The listing builds one solid part. Answer for the finished solid, in the listing's coordinates (mm). Coordinates: 2 decimals unless noted, no trailing zeros. Order: outer loops, then holes, each group sorted by start corner. A loop starts at its lowest first (then second) coordinate and runs counter-clockwise, first axis right, second up. Notation, with made-up numbers: (9.25, -30) -> (51.25, -30) arc R12 ccw to (51.25, -16) -> close; hole circle Ø8 at (27.5, 55.25). An arc over 180 degrees is marked (long way). Write each question's results on one line, items separated by ' | '. Start each with the question number.
(1) The part is cut by section C-C, the plane x = -32. Give the vertices of the cut face in (y, z).
(2) The part is cut by section A-A, the plane z = 57. Give the vertices of the cut face in (x, y).
(3) Given pin 1 (1.5 mm diameter, centred on x = 1.5, y = -4.5, fed in from -Z); pin 2 (1.5 mm diameter, centred on x = -1.5, y = -4, fed in from +Z); pin 3 (2 mm diameter, centred on x = -16.5, z = 46.5, fed in from -Y); pin 4 (4 mm diameter, centred on y = -5.5, z = 26, fed in from +X), each flat-ended and moving along its own axis, determine where each tip first touches the part or whether it passes through.
(4) Determine the mould class of faces 1 (the face through (-30.54, -6.26, 34.89)), 2 (the face through (-24.83, -6.26, 35)), 3 (the face through (30.966, -6.261, 33.991)), 4 (the face through (24.365, -6.261, 35.917)) for opening direction X: +X half, -X half, draft (parallel to the pull), parting line (faces both ways), or undercut.
(5) The part is cut by section D-D, the plane x = 21. Give the vertices of the cut face in (y, z).
(6) Straight lines are drawn through the part: L1, parallel to X at y = -6.25, z = 54; L2, parallel to X at y = -11, z = 55.5; L3, parallel to Z at x = -17, y = -9.75. For each, find the intervals that lie inside material, in ascending order.
(7) The part is cut by section B-B, the plane z = 29.5. Give the vertices of the cut face in (x, y).
```python
from build123d import *

# Parameters (mm, degrees)
F1_DEPTH = 12.7
F2_R     = 15.24
F3_R     = 5.08


with BuildPart() as f1:
    # F0 (on Front) → F1 (new body)
    with BuildSketch(Plane.XZ):
        with BuildLine():
            ThreePointArc((41.717369, 0.82729), (26.878905, 42.014486), (0, 76.570086))
            ThreePointArc((0, 76.570086), (-26.878905, 42.014486), (-41.717369, 0.82729))
            Line((-41.717369, 0.82729), (-36.542559, 0.82729))
            ThreePointArc((-36.542559, 0.82729), (-23.349687, 37.863578), (0, 69.494744))
            ThreePointArc((0, 69.494744), (23.349687, 37.863578), (36.542559, 0.82729))
            Line((36.542559, 0.82729), (41.717369, 0.82729))
        make_face()
    extrude(amount=F1_DEPTH)

    # F2
    f2_edges = [f1.edges().sort_by_distance(p)[0] for p in [
        (0, -6.35, 76.570086),
    ]]
    fillet(f2_edges, radius=F2_R)

    # F3
    f3_edges = [f1.edges().sort_by_distance(p)[0] for p in [
        (0, -6.35, 69.494744),
    ]]
    fillet(f3_edges, radius=F3_R)

    # F5 (on offset) → F6 (revolve)
    with BuildSketch(Plane.XZ.offset(6.35)):
        with BuildLine():
            Line((39.129964, 0.82729), (37.655077, 0.82729))
            add(Edge.make_bspline(
                [(37.655077, 0.82729), (36.695255, -4.188608), (37.93704, -9.83515), (39.129964, -12.974122)],
                knots=[0, 0, 0, 0, 13.879995, 13.879995, 13.879995, 13.879995], degree=3))
            Line((39.129964, -12.974122), (39.129964, 0.82729))
        make_face()
    revolve(axis=Axis((39.129964, -6.35, -6.073416), (0, 0, 1)))

    # F5 (on offset) → F7 (revolve)
    with BuildSketch(Plane.XZ.offset(6.35)):
        with BuildLine():
            Line((-39.129964, 0.82729), (-40.604852, 0.82729))
            add(Edge.make_bspline(
                [(-40.604852, 0.82729), (-41.564673, -4.188608), (-40.322889, -9.83515), (-39.129964, -12.974122)],
                knots=[0, 0, 0, 0, 13.879995, 13.879995, 13.879995, 13.879995], degree=3))
            Line((-39.129964, -12.974122), (-39.129964, 0.82729))
        make_face()
    revolve(axis=Axis((-39.129964, -6.35, -6.073416), (0, 0, 1)))


solid = f1.part
```
Established:
1) outline: (-12.7, 17.84) -> (0, 17.84) -> (0, 31.74) -> (-12.7, 31.74) -> close
2) outline: (-17.33, -12.7) -> (-10.98, -12.7) -> (-10.98, 0) -> (-17.33, 0) -> close; (10.98, -12.7) -> (17.33, -12.7) -> (17.33, 0) -> (10.98, 0) -> close
3) pin 1: stops at z = 66.7 | pin 2: stops at z = 69.66 | pin 3: passes through | pin 4: stops at x = 35.19
4) face 1: -X half | face 2: undercut | face 3: +X half | face 4: undercut
5) outline: (-12.7, 42.09) -> (0, 42.09) -> (0, 51.73) -> (-12.7, 51.73) -> close
6) L1: x = -19.46 to -13.23, 13.23 to 19.46 | L2: x = -18.41 to -12.12, 12.12 to 18.41 | L3: z = 48.57 to 57.45
7) outline: (-32.98, -12.7) -> (-27.44, -12.7) -> (-27.44, 0) -> (-32.98, 0) -> close; (27.44, -12.7) -> (32.98, -12.7) -> (32.98, 0) -> (27.44, 0) -> close
